The model under review builds one solid part; all positions refer to its coordinate system, in mm. Face numbers are marked on the shaded views. A direction names the side the tool comes from. Round coordinates to 2 decimals unless told otherwise and drop trailing zeros. Write each loop counter-clockwise with the first axis right and the second up, starting at its lowest first coordinate (ties: lowest second). Pieces come first, ordered by that corner, then holes.
Item 1: Clearance check with flat-ended pins moving along their axes: pin 1 Ø1.2 at (x, y) = (-40, 25) entering from -Z; pin 2 Ø2.5 at (x, y) = (-30, 16.34) entering from -Z; pin 3 Ø3 at (x, y) = (-10, 25) entering from +Z; pin 4 Ø3 at (x, y) = (-25, 25) entering from -Z. State where each tip first meets the part, or that it passes through.
Item 2: Add section D-D (y = 25). State how many separate pieces and enclosed holes the cut face has, plus the area to 3 significant figures.
Item 3: Add section C-C (x = -12.5). Give the boundary of the cut face in (y, z), plus the area to 3 significant figures.
Item 4: Machinability: for the marked faces 1 and 2, which of the approach directions +Z, -Z, +X, -X, +Y, -Y give a long, thin tool a straight path to every point of the face, cutting with its end or side? Answer none if there is none.
Item 5: To check wall thickness, follow L1, parallel to Y at x = -30, z = 0.9; L2, parallel to Y at x = -22.5, z = 0.9; L3, parallel to Y at x = -27.5, z = 1.15. State the ranges of each line that lie inside material, in increasing order.
Item 6: Add section A-A (z = 1.6). Give the boundary of the cut face in (x, y).
Item 7: Add section B-B (x = -20). Give the boundary of the cut face in (y, z), plus the area to 3 significant figures.
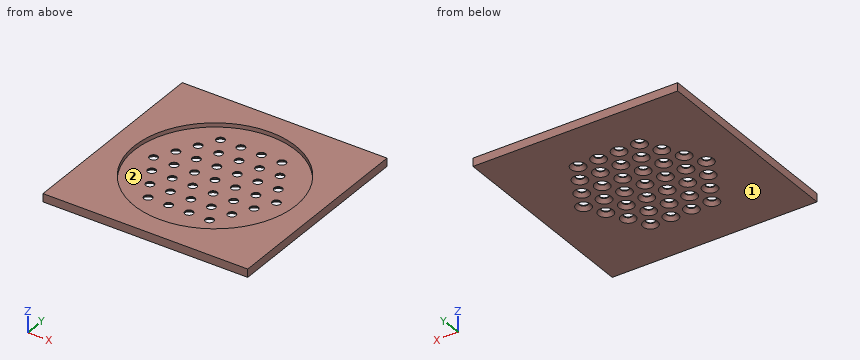
```python
from build123d import *

# Parameters (mm, degrees)
SKETCH_1_W             = 50
SKETCH_1_H             = 50
EXTRUDE_1_DEPTH        = 2
SKETCH_2_R             = 1
CUT_EXTRUDE_1849_DEPTH = 71.738956735
SKETCH_3_R             = 19.75
CUT_EXTRUDE_2321_DEPTH = 1
CHAMFER_1_SIZE         = 0.8


with BuildPart() as part:
    # Эскиз1 → Бобышка-Вытянуть1 (new body)
    with BuildSketch(Plane(origin=(0, 66.754264805, 0), x_dir=(-1, 0, 0), z_dir=(0, 0, 1))):
        with Locations((25, 41.754264805)):
            Rectangle(SKETCH_1_W, SKETCH_1_H)
    extrude(amount=EXTRUDE_1_DEPTH)

    # Эскиз2 → Cut-Extrude 1849 (cut, through all)
    with BuildSketch(Plane.XY.offset(2)):
        with Locations((-25, 25)):
            Circle(SKETCH_2_R)
        with Locations((-20, 25)):
            Circle(SKETCH_2_R)
        with Locations((-15, 25)):
            Circle(SKETCH_2_R)
        with Locations((-10, 25)):
            Circle(SKETCH_2_R)
        with Locations((-22.5, 20.669872981)):
            Circle(SKETCH_2_R)
        with Locations((-20, 16.339745962)):
            Circle(SKETCH_2_R)
        with Locations((-17.5, 12.009618943)):
            Circle(SKETCH_2_R)
        with Locations((-27.5, 20.669872981)):
            Circle(SKETCH_2_R)
        with Locations((-30, 16.339745962)):
            Circle(SKETCH_2_R)
        with Locations((-32.5, 12.009618943)):
            Circle(SKETCH_2_R)
        with Locations((-30, 25)):
            Circle(SKETCH_2_R)
        with Locations((-35, 25)):
            Circle(SKETCH_2_R)
        with Locations((-40, 25)):
            Circle(SKETCH_2_R)
        with Locations((-27.5, 29.330127019)):
            Circle(SKETCH_2_R)
        with Locations((-30, 33.660254038)):
            Circle(SKETCH_2_R)
        with Locations((-32.5, 37.990381057)):
            Circle(SKETCH_2_R)
        with Locations((-22.5, 29.330127019)):
            Circle(SKETCH_2_R)
        with Locations((-20, 33.660254038)):
            Circle(SKETCH_2_R)
        with Locations((-17.5, 37.990381057)):
            Circle(SKETCH_2_R)
        with Locations((-25, 16.339745962)):
            Circle(SKETCH_2_R)
        with Locations((-27.5, 12.009618943)):
            Circle(SKETCH_2_R)
        with Locations((-22.5, 12.009618943)):
            Circle(SKETCH_2_R)
        with Locations((-32.5, 20.669872981)):
            Circle(SKETCH_2_R)
        with Locations((-37.5, 20.669872981)):
            Circle(SKETCH_2_R)
        with Locations((-35, 16.339745962)):
            Circle(SKETCH_2_R)
        with Locations((-32.5, 29.330127019)):
            Circle(SKETCH_2_R)
        with Locations((-35, 33.660254038)):
            Circle(SKETCH_2_R)
        with Locations((-37.5, 29.330127019)):
            Circle(SKETCH_2_R)
        with Locations((-25, 33.660254038)):
            Circle(SKETCH_2_R)
        with Locations((-22.5, 37.990381057)):
            Circle(SKETCH_2_R)
        with Locations((-27.5, 37.990381057)):
            Circle(SKETCH_2_R)
        with Locations((-17.5, 29.330127019)):
            Circle(SKETCH_2_R)
        with Locations((-12.5, 29.330127019)):
            Circle(SKETCH_2_R)
        with Locations((-15, 33.660254038)):
            Circle(SKETCH_2_R)
        with Locations((-17.5, 20.669872981)):
            Circle(SKETCH_2_R)
        with Locations((-15, 16.339745962)):
            Circle(SKETCH_2_R)
        with Locations((-12.5, 20.669872981)):
            Circle(SKETCH_2_R)
    extrude(amount=-CUT_EXTRUDE_1849_DEPTH, mode=Mode.SUBTRACT)

    # Эскиз3 → Cut-Extrude 2321 (cut)
    with BuildSketch(Plane.XY.offset(2)):
        with Locations((-25, 25)):
            Circle(SKETCH_3_R)
    extrude(amount=-CUT_EXTRUDE_2321_DEPTH, mode=Mode.SUBTRACT)

    # Фаска1
    chamfer_1_edges = [part.edges().sort_by_distance(p)[0] for p in [
        (-33.5, 12.009618943, 0),
        (-31, 25, 0),
        (-36, 25, 0),
        (-41, 25, 0),
        (-23.5, 29.330127019, 0),
        (-33.5, 37.990381057, 0),
        (-31, 33.660254038, 0),
        (-28.5, 29.330127019, 0),
        (-13.5, 20.669872981, 0),
        (-16, 16.339745962, 0),
        (-18.5, 20.669872981, 0),
        (-16, 33.660254038, 0),
        (-26, 25, 0),
        (-36, 16.339745962, 0),
        (-38.5, 20.669872981, 0),
        (-33.5, 20.669872981, 0),
        (-23.5, 12.009618943, 0),
        (-28.5, 12.009618943, 0),
        (-26, 16.339745962, 0),
        (-18.5, 37.990381057, 0),
        (-21, 33.660254038, 0),
        (-13.5, 29.330127019, 0),
        (-18.5, 29.330127019, 0),
        (-28.5, 37.990381057, 0),
        (-23.5, 37.990381057, 0),
        (-33.5, 29.330127019, 0),
        (-36, 33.660254038, 0),
        (-38.5, 29.330127019, 0),
        (-26, 33.660254038, 0),
        (-31, 16.339745962, 0),
        (-28.5, 20.669872981, 0),
        (-18.5, 12.009618943, 0),
        (-21, 16.339745962, 0),
        (-21, 25, 0),
        (-16, 25, 0),
        (-11, 25, 0),
        (-23.5, 20.669872981, 0),
    ]]
    chamfer(chamfer_1_edges, length=CHAMFER_1_SIZE)


solid = part.part
```
Numbers:
1. pin 1: passes through
1. pin 2: stops at z = 0.55
1. pin 3: stops at z = 1
1. pin 4: stops at z = 0.3
2. separate pieces: 8
2. enclosed holes: 0
2. area: 42.0 mm2
3. outline: (0, 0) - (18.87, 0) - (19.67, 0.8) - (19.67, 1) - (9.71, 1) - (9.71, 2) - (0, 2) - close; (21.67, 0.8) - (22.47, 0) - (27.53, 0) - (28.33, 0.8) - (28.33, 1) - (21.67, 1) - close; (30.33, 0.8) - (31.13, 0) - (50, 0) - (50, 2) - (40.29, 2) - (40.29, 1) - (30.33, 1) - close
3. area: 64.1 mm2
4. face 1: -Z, +X, -X, +Y, -Y
4. face 2: +Z
5. L1: y = 0 to 15.34, 17.34 to 24, 26 to 32.66, 34.66 to 50
5. L2: y = 0 to 11.01, 13.01 to 19.67, 21.67 to 28.33, 30.33 to 36.99, 38.99 to 50
5. L3: y = 0 to 5.41, 44.59 to 50
6. outline: (-50, 0) - (0, 0) - (0, 50) - (-50, 50) - close; hole circle Ø39.5 at (-25, 25)
7. outline: (0, 0) - (14.54, 0) - (15.34, 0.8) - (15.34, 1) - (5.89, 1) - (5.89, 2) - (0, 2) - close; (17.34, 0.8) - (18.14, 0) - (23.2, 0) - (24, 0.8) - (24, 1) - (17.34, 1) - close; (26, 0.8) - (26.8, 0) - (31.86, 0) - (32.66, 0.8) - (32.66, 1) - (26, 1) - close; (34.66, 0.8) - (35.46, 0) - (50, 0) - (50, 2) - (44.11, 2) - (44.11, 1) - (34.66, 1) - close
7. area: 53.9 mm2
